from build123d import *

# Parameters (mm, degrees)
SKETCH1_W           = 60
SKETCH1_H           = 80
BOSS_EXTRUDE1_DEPTH = 3
SKETCH2_R           = 2.5
CUT_EXTRUDE1_DEPTH  = 3
SKETCH3_R           = 1.5
CUT_EXTRUDE2_DEPTH  = 3


with BuildPart() as part:
    # Sketch1 → Boss-Extrude1 (new body)
    with BuildSketch(Plane.XY):
        Rectangle(SKETCH1_W, SKETCH1_H)
    extrude(amount=-BOSS_EXTRUDE1_DEPTH)

    # Sketch2 → Cut-Extrude1 (cut)
    with BuildSketch(Plane.XY):
        with Locations((-25, 35)):
            Circle(SKETCH2_R)
        with Locations((-25, -35)):
            Circle(SKETCH2_R)
        with Locations((25, -35)):
            Circle(SKETCH2_R)
        with Locations((25, 35)):
            Circle(SKETCH2_R)
    extrude(amount=-CUT_EXTRUDE1_DEPTH, mode=Mode.SUBTRACT)

    # Sketch3 → Cut-Extrude2 (cut)
    with BuildSketch(Plane.XY):
        with Locations((-18.5, 29)):
            Circle(SKETCH3_R)
        with Locations((-18.5, -1.48)):
            Circle(SKETCH3_R)
        with Locations((17.06, -1.48)):
            Circle(SKETCH3_R)
    extrude(amount=-CUT_EXTRUDE2_DEPTH, mode=Mode.SUBTRACT)


solid = part.part
Input: part model. Units: mm. Frame: model coordinates. Coordinates: 2 decimals unless noted, no trailing zeros. Loops run counter-clockwise (first coordinate to the right, second up) from the corner with the lowest first, then second, coordinate; pieces in that order, holes last.
(1) First-contact query: pin 1 Ø2.5 at (x, y) = (17.06, -1.48) entering from -Z. Flat tip, straight axial feed; report the tip coordinate or a pass-through.
(2) Section B-B on z = -2.15. Return the cut outline in (x, y).
(3) Section D-D on x = 17.06. Return the cut outline in (y, z).
(4) Material intervals for probe 1 along Y at (x, z) = (25, -0.85); probe 2 along X at (y, z) = (35.5, -0.9); probe 3 along Y at (x, z) = (17.06, -2.2), sorted ascending.
(5) Section C-C on x = -18.5. Return the cut outline in (y, z).
(6) Section A-A on y = 29. Return the cut outline in (x, z).
(7) Pull-direction query (X, two-part tool) for faces 1 (the face through (23.16, 36.69, -1.48)), 2 (the face through (-26.84, -33.31, -1.48)), 3 (the face through (30, -1, -1)), 4 (the face through (0, 1, 0)); classes: released by +X, released by -X, zero draft, split by the parting line, or undercut.
Data:
1. pin 1: passes through
2. outline: (-30, -40) - (30, -40) - (30, 40) - (-30, 40) - close; hole circle Ø5 at (-25, -35); hole circle Ø5 at (-25, 35); hole circle Ø3 at (-18.5, -1.48); hole circle Ø3 at (-18.5, 29); hole circle Ø3 at (17.06, -1.48); hole circle Ø5 at (25, -35); hole circle Ø5 at (25, 35)
3. outline: (-40, -3) - (-2.98, -3) - (-2.98, 0) - (-40, 0) - close; (0.02, -3) - (40, -3) - (40, 0) - (0.02, 0) - close
4. probe 1: y = -40 to -37.5, -32.5 to 32.5, 37.5 to 40
4. probe 2: x = -30 to -27.45, -22.55 to 22.55, 27.45 to 30
4. probe 3: y = -40 to -2.98, 0.02 to 40
5. outline: (-40, -3) - (-2.98, -3) - (-2.98, 0) - (-40, 0) - close; (0.02, -3) - (27.5, -3) - (27.5, 0) - (0.02, 0) - close; (30.5, -3) - (40, -3) - (40, 0) - (30.5, 0) - close
6. outline: (-30, -3) - (-20, -3) - (-20, 0) - (-30, 0) - close; (-17, -3) - (30, -3) - (30, 0) - (-17, 0) - close
7. face 1: undercut
7. face 2: undercut
7. face 3: released by +X
7. face 4: zero draft
